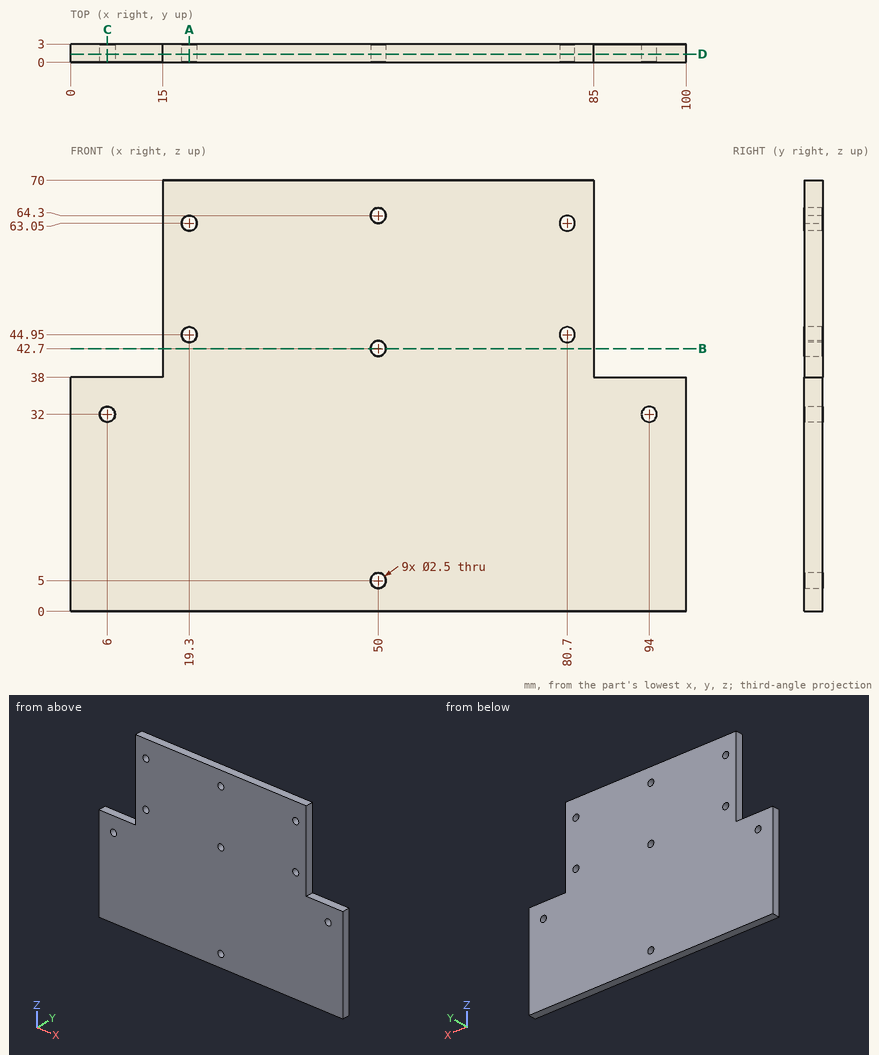
Answer from the drawing. Dimensions are ordinates in mm from the lowest x, y and z of the part. Round coordinates to 2 decimals unless told otherwise and drop trailing zeros. Write each loop counter-clockwise with the first axis right and the second up, starting at its lowest first coordinate (ties: lowest second). Pieces come first, ordered by that corner, then holes. Notation, with made-up numbers: (16.5, 60.25) -> (68.5, 60.25) arc R33 ccw to (68.5, 93.25) -> close; hole circle Ø1 at (28, 35). An arc over 180 degrees is marked (long way). Write each question's results on one line, items separated by ' | '.
1) Consider line 1 along Z through (x, y) = (80.7, 1); line 2 along X through (y, z) = (2.55, 45); line 3 along X through (y, z) = (1.85, 32.5). Determine where each line is inside the solid, lowest interval first. Write a range as [from, to].
Findings:
line 1: z = [0, 43.7], [46.2, 61.8], [64.3, 70] | line 2: x = [15, 18.05], [20.55, 79.45], [81.95, 85] | line 3: x = [0, 4.85], [7.15, 92.85], [95.15, 100]
2) The part is cut by section A-A (x = 19.3). Write down the section's boundary in (y, z).
Findings:
outline: (0, 0) -> (3, 0) -> (3, 43.7) -> (0, 43.7) -> close; (0, 46.2) -> (3, 46.2) -> (3, 61.8) -> (0, 61.8) -> close; (0, 64.3) -> (3, 64.3) -> (3, 70) -> (0, 70) -> close
3) The part is cut by section B-B (z = 42.7). Write down the section's boundary in (x, y).
Findings:
outline: (15, 0) -> (48.75, 0) -> (48.75, 3) -> (15, 3) -> close; (51.25, 0) -> (85, 0) -> (85, 3) -> (51.25, 3) -> close
4) The part is cut by section D-D (y = 1.35). State how many separate pieces and enclosed holes the cut face has, and give its area (3 significant figures).
Findings:
separate pieces: 1 | enclosed holes: 9 | area: 6,000 mm²
5) The part is cut by section C-C (x = 6). Write down the section's boundary in (y, z), and give its area (4 significant figures).
Findings:
outline: (0, 0) -> (3, 0) -> (3, 30.75) -> (0, 30.75) -> close; (0, 33.25) -> (3, 33.25) -> (3, 38) -> (0, 38) -> close | area: 106.5 mm²
6) Flat-ended cylindrical pins translate along their axes: pin 1 (1.5 mm diameter, centred on x = 19.3, z = 63.05, fed in from +Y); pin 2 (0.9 mm diameter, centred on y = 1.5, z = 53.5, fed in from +X); pin 3 (1.5 mm diameter, centred on x = 8, y = 1, fed in from +Z). Find the tip coordinate at first contact, or state that the pin passes through.
Findings:
pin 1: passes through | pin 2: stops at x = 85 | pin 3: stops at z = 38
